Could you check a few things on this model? Use its own coordinates, in mm. Face numbers are marked on the shaded views. A direction names the side the tool comes from. Give positions to 0.01 mm unless a question says otherwise; leave off trailing zeros. Loops run counter-clockwise (first coordinate to the right, second up) from the corner with the lowest first, then second, coordinate; pieces in that order, holes last. Notation, with made-up numbers: M 18,61.25 L 29,61.25 A25 cw 29,83.25 Z; hole C 64.25,65.25 d3. An arc over 180 degrees is marked long. Return JSON: item names as keys, results as strings. Group by question number.
1. If we mould it in two halves opening along Y, with no side actions, what happens to the marked faces 5, 6 and 7? For each: +Y half, -Y half, draft (parallel to the pull), parting line (faces both ways), or undercut.
2. If we section it at C-C (y = -16.5): Write out the boundary of the cut face in (x, z).
3. Please list where these lines run through material, in increasing order: line 1 (Y direction, x = 0, z = 25.5); line 2 (Z direction, x = 39, y = 52); line 3 (Y direction, x = 2.5, z = 4).
4. For pin 1 (1.3 mm diameter, centred on y = 14.5, z = 22.5, fed in from -X); pin 2 (1.5 mm diameter, centred on x = 25.5, y = 56.5, fed in from +Z); pin 3 (1 mm diameter, centred on y = -23.5, z = 33.5, fed in from -X), each with a flat end and sliding along its axis, tell me the tip position at first contact or that it passes through.
5. If we section it at D-D (y = 38): Write out the boundary of the cut face in (x, z).
6. If we section it at A-A (x = 0): Write out the boundary of the cut face in (y, z), plus the area to 3 significant figures.
7. For the marked faces 1, 2, 3 and 4, which set-ups out of +Z, -Z, +X, -X, +Y, -Y let a thin tool reach every point of the face, with its end or its side?
8. If we section it at B-B (z = 36): Write out the boundary of the cut face in (x, y).
```python
from build123d import *

# Parameters (mm, degrees)
BOSS_EXTRUDE1_DEPTH = 20
SKETCH3_R           = 30
BOSS_EXTRUDE2_DEPTH = 20
CUT_EXTRUDE1_DEPTH  = 127.092159028


with BuildPart() as part:
    # Sketch1 → Boss-Extrude1 (new body)
    with BuildSketch(Plane.XY):
        with BuildLine():
            Line((6.339757092, 74.731569501), (2.843370149, 84.549554706))
            Line((2.843370149, 84.549554706), (-2.843370149, 84.549554706))
            Line((-2.843370149, 84.549554706), (-6.339757092, 74.731569501))
            ThreePointArc((-6.339757092, 74.731569501), (-9.399992517, 74.408602599), (-12.444403622, 73.960373299))
            Line((-12.444403622, 73.960373299), (-18.272578772, 82.600392371))
            Line((-18.272578772, 82.600392371), (-23.780659667, 81.186157568))
            Line((-23.780659667, 81.186157568), (-24.725567552, 70.807106347))
            ThreePointArc((-24.725567552, 70.807106347), (-27.609341451, 69.733236442), (-30.446636689, 68.541974836))
            Line((-30.446636689, 68.541974836), (-38.240394368, 75.4611436))
            Line((-38.240394368, 75.4611436), (-43.223722879, 72.721535567))
            Line((-43.223722879, 72.721535567), (-41.557779668, 62.433572291))
            ThreePointArc((-41.557779668, 62.433572291), (-44.083893922, 60.676274578), (-46.535795597, 58.816832014))
            Line((-46.535795597, 58.816832014), (-55.805425347, 63.58039365))
            Line((-55.805425347, 63.58039365), (-59.950880617, 59.687552036))
            Line((-59.950880617, 59.687552036), (-55.778763649, 50.137107274))
            ThreePointArc((-55.778763649, 50.137107274), (-57.788493208, 47.806799231), (-59.700939322, 45.396011323))
            Line((-59.700939322, 45.396011323), (-69.863996213, 47.704653735))
            Line((-69.863996213, 47.704653735), (-72.911104041, 42.903180095))
            Line((-72.911104041, 42.903180095), (-66.49496277, 34.690343415))
            ThreePointArc((-66.49496277, 34.690343415), (-67.862028935, 31.933446867), (-69.114853465, 29.122792286))
            Line((-69.114853465, 29.122792286), (-79.532755256, 28.83145498))
            Line((-79.532755256, 28.83145498), (-81.290054651, 23.423043562))
            Line((-81.290054651, 23.423043562), (-73.033038828, 17.063857698))
            ThreePointArc((-73.033038828, 17.063857698), (-73.671543805, 14.053598594), (-74.186027177, 11.019681104))
            Line((-74.186027177, 11.019681104), (-84.204178785, 8.146669874))
            Line((-84.204178785, 8.146669874), (-84.561252162, 2.471151058))
            Line((-84.561252162, 2.471151058), (-74.98218046, -1.634812956))
            ThreePointArc((-74.98218046, -1.634812956), (-74.852004632, -4.709288965), (-74.595819965, -7.77583717))
            Line((-74.595819965, -7.77583717), (-83.584744079, -13.050000462))
            Line((-83.584744079, -13.050000462), (-82.519155206, -18.636012955))
            Line((-82.519155206, -18.636012955), (-72.219915929, -20.230762298))
            ThreePointArc((-72.219915929, -20.230762298), (-71.329238722, -23.176274578), (-70.318483041, -26.082770996))
            Line((-70.318483041, -26.082770996), (-77.7133725, -33.426691274))
            Line((-77.7133725, -33.426691274), (-75.292076244, -38.572207736))
            Line((-75.292076244, -38.572207736), (-64.919808474, -37.555538443))
            ThreePointArc((-64.919808474, -37.555538443), (-63.324594413, -40.187009623), (-61.622777213, -42.750828396))
            Line((-61.622777213, -42.750828396), (-66.958983917, -51.703060138))
            Line((-66.958983917, -51.703060138), (-63.334119227, -56.084768847))
            Line((-63.334119227, -56.084768847), (-53.540550694, -52.520561987))
            ThreePointArc((-53.540550694, -52.520561987), (-51.341032945, -54.672647057), (-49.055085661, -56.73269402))
            Line((-49.055085661, -56.73269402), (-51.997316116, -66.730735583))
            Line((-51.997316116, -66.730735583), (-47.396646572, -70.073317665))
            Line((-47.396646572, -70.073317665), (-38.797143205, -64.185525464))
            ThreePointArc((-38.797143205, -64.185525464), (-36.131525558, -65.723001003), (-33.405082664, -67.149835831))
            Line((-33.405082664, -67.149835831), (-33.768465712, -77.565473494))
            Line((-33.768465712, -77.565473494), (-28.4810683, -79.658902223))
            Line((-28.4810683, -79.658902223), (-21.615968523, -71.817476319))
            ThreePointArc((-21.615968523, -71.817476319), (-18.651741537, -72.643737085), (-15.656115469, -73.347706497))
            Line((-15.656115469, -73.347706497), (-13.417818414, -83.526487439))
            Line((-13.417818414, -83.526487439), (-7.775919761, -84.239224989))
            Line((-7.775919761, -84.239224989), (-3.076583041, -74.93687101))
            ThreePointArc((-3.076583041, -74.93687101), (0, -75), (3.076583041, -74.93687101))
            Line((3.076583041, -74.93687101), (7.775919761, -84.239224989))
            Line((7.775919761, -84.239224989), (13.417818414, -83.526487439))
            Line((13.417818414, -83.526487439), (15.656115469, -73.347706497))
            ThreePointArc((15.656115469, -73.347706497), (18.651741537, -72.643737085), (21.615968523, -71.817476319))
            Line((21.615968523, -71.817476319), (28.4810683, -79.658902223))
            Line((28.4810683, -79.658902223), (33.768465712, -77.565473494))
            Line((33.768465712, -77.565473494), (33.405082664, -67.149835831))
            ThreePointArc((33.405082664, -67.149835831), (36.131525558, -65.723001003), (38.797143205, -64.185525464))
            Line((38.797143205, -64.185525464), (47.396646572, -70.073317665))
            Line((47.396646572, -70.073317665), (51.997316116, -66.730735583))
            Line((51.997316116, -66.730735583), (49.055085661, -56.73269402))
            ThreePointArc((49.055085661, -56.73269402), (51.341032945, -54.672647057), (53.540550694, -52.520561987))
            Line((53.540550694, -52.520561987), (63.334119227, -56.084768847))
            Line((63.334119227, -56.084768847), (66.958983917, -51.703060138))
            Line((66.958983917, -51.703060138), (61.622777213, -42.750828396))
            ThreePointArc((61.622777213, -42.750828396), (63.324594413, -40.187009623), (64.919808474, -37.555538443))
            Line((64.919808474, -37.555538443), (75.292076244, -38.572207736))
            Line((75.292076244, -38.572207736), (77.7133725, -33.426691274))
            Line((77.7133725, -33.426691274), (70.318483041, -26.082770996))
            ThreePointArc((70.318483041, -26.082770996), (71.329238722, -23.176274578), (72.219915929, -20.230762298))
            Line((72.219915929, -20.230762298), (82.519155206, -18.636012955))
            Line((82.519155206, -18.636012955), (83.584744079, -13.050000462))
            Line((83.584744079, -13.050000462), (74.595819965, -7.77583717))
            ThreePointArc((74.595819965, -7.77583717), (74.852004632, -4.709288965), (74.98218046, -1.634812956))
            Line((74.98218046, -1.634812956), (84.561252162, 2.471151058))
            Line((84.561252162, 2.471151058), (84.204178785, 8.146669874))
            Line((84.204178785, 8.146669874), (74.186027177, 11.019681104))
            ThreePointArc((74.186027177, 11.019681104), (73.671543805, 14.053598594), (73.033038828, 17.063857698))
            Line((73.033038828, 17.063857698), (81.290054651, 23.423043562))
            Line((81.290054651, 23.423043562), (79.532755256, 28.83145498))
            Line((79.532755256, 28.83145498), (69.114853465, 29.122792286))
            ThreePointArc((69.114853465, 29.122792286), (67.862028935, 31.933446867), (66.49496277, 34.690343415))
            Line((66.49496277, 34.690343415), (72.911104041, 42.903180095))
            Line((72.911104041, 42.903180095), (69.863996213, 47.704653735))
            Line((69.863996213, 47.704653735), (59.700939322, 45.396011323))
            ThreePointArc((59.700939322, 45.396011323), (57.788493208, 47.806799231), (55.778763649, 50.137107274))
            Line((55.778763649, 50.137107274), (59.950880617, 59.687552036))
            Line((59.950880617, 59.687552036), (55.805425347, 63.58039365))
            Line((55.805425347, 63.58039365), (46.535795597, 58.816832014))
            ThreePointArc((46.535795597, 58.816832014), (44.083893922, 60.676274578), (41.557779668, 62.433572291))
            Line((41.557779668, 62.433572291), (43.223722879, 72.721535567))
            Line((43.223722879, 72.721535567), (38.240394368, 75.4611436))
            Line((38.240394368, 75.4611436), (30.446636689, 68.541974836))
            ThreePointArc((30.446636689, 68.541974836), (27.609341451, 69.733236442), (24.725567552, 70.807106347))
            Line((24.725567552, 70.807106347), (23.780659667, 81.186157568))
            Line((23.780659667, 81.186157568), (18.272578772, 82.600392371))
            Line((18.272578772, 82.600392371), (12.444403622, 73.960373299))
            ThreePointArc((12.444403622, 73.960373299), (9.399992517, 74.408602599), (6.339757092, 74.731569501))
        make_face()
    extrude(amount=BOSS_EXTRUDE1_DEPTH)

    # Sketch3 → Boss-Extrude2 (add)
    with BuildSketch(Plane.XY.offset(20)):
        Circle(SKETCH3_R)
    extrude(amount=BOSS_EXTRUDE2_DEPTH)

    # Sketch4 → Cut-Extrude1 (cut, through all)
    with BuildSketch(Plane.XY.offset(40)):
        with BuildLine():
            Line((-6, 16), (6, 16))
            Line((6, 16), (6, 11.532562595))
            ThreePointArc((6, 11.532562595), (0, -13), (-6, 11.532562595))
            Line((-6, 11.532562595), (-6, 16))
        make_face()
    extrude(amount=-CUT_EXTRUDE1_DEPTH, mode=Mode.SUBTRACT)


solid = part.part
```
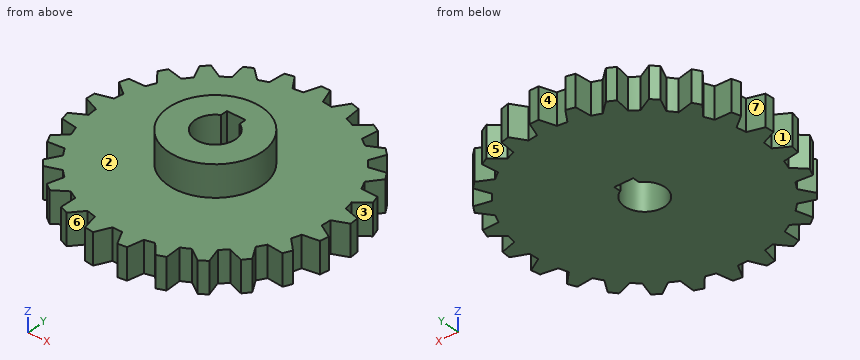
Answer:
{
 "1": {"face 5": "+Y half", "face 6": "-Y half", "face 7": "undercut"},
 "2": {"outline": "M -82.93,0 L 82.93,0 L 82.93,20 L 25.05,20 L 25.05,40 L -25.05,40 L -25.05,20 L -82.93,20 Z"},
 "3": {"line 1": "y = -30 to -13, 16 to 30", "line 2": "z = 0 to 20", "line 3": "y = -74.96 to -12.76, 16 to 84.55"},
 "4": {"pin 1": "stops at x = -26.61", "pin 2": "stops at z = 20", "pin 3": "stops at x = -19.26"},
 "5": {"outline": "M -69.08,0 L 69.08,0 L 69.08,20 L -69.08,20 Z"},
 "6": {"outline": "M -75,0 L -13,0 L -13,40 L -30,40 L -30,20 L -75,20 Z; M 16,0 L 84.55,0 L 84.55,20 L 30,20 L 30,40 L 16,40 Z", "area": "3,230 mm²"},
 "7": {"face 1": "+Z, -Z, -X", "face 2": "+Z", "face 3": "+Z, -Z, +X", "face 4": "+Z, -Z, +Y"},
 "8": {"outline": "C 0,0 d60; hole M -6,11.53 A13 ccw long 6,11.53 L 6,16 L -6,16 Z"}
}
